Can you work these out from the model? Positions are in its coordinate system, mm. A direction names the side the tool comes from. Coordinates: 2 decimals unless noted, no trailing zeros. Order: outer loops, then holes, each group sorted by start corner. A loop starts at its lowest first (then second) coordinate and runs counter-clockwise, first axis right, second up. Notation, with made-up numbers: (48, 85.5) -> (89, 85.5) arc R27 ccw to (89, 103.5) -> close; hole circle Ø1 at (-9.5, 3). An arc over 180 degrees is marked (long way). Answer in a Markdown table with one row per item. Add a question column.
1. On a 3-axis mill with a long thin cutter (end or side, diameter ignored), from which of +Z, -Z, +X, -X, +Y, -Y can I reach the whole of each face in a straight line? I mean faces 1 (the face through (-160, -1, 65)), 2 (the face through (-2, 85, 65)), 3 (the face through (-155.49, -80.72, 65.35)), 4 (the face through (160, -1, 65)). Say none if no direction works.
2. If I drill on line 1 along X through (y, z) = (-57.5, 39.5); line 2 along Z through (x, y) = (225, 83); line 3 along Y through (x, z) = (17, 62), over which ranges is the centre line in solid material (lowest first)? Write a range as [from, to].
3. Will these pins go through, and if not, where does the flat tip stop? pin 1 (4 mm diameter, centred on x = 47.5, y = -89.5, fed in from +Z); pin 2 (15 mm diameter, centred on y = 32, z = 63.5, fed in from +X); pin 3 (8 mm diameter, centred on x = 159.5, z = 72.5, fed in from -Y).
4. Imagine slicing it at A-A on y = -1. Write out the boundary of the cut face in (x, z), plus the area to 3 significant figures.
5. Imagine slicing it at C-C on x = 75. Write out the boundary of the cut face in (y, z), plus the area to 3 significant figures.
6. Imagine slicing it at B-B on z = 57.5. Write out the boundary of the cut face in (x, y), plus the area to 3 significant figures.
7. Imagine slicing it at D-D on x = 214. Write out the boundary of the cut face in (y, z).
from build123d import *

# Parameters (mm, degrees)
F0_W     = 500
F0_H     = 250
F1_DEPTH = 25
F2_W     = 320
F2_H     = 170
F3_DEPTH = 80
F4_R     = 15


with BuildPart() as f1:
    # F0 (on Top) → F1 (new body, symmetric)
    with BuildSketch(Plane.XY):
        Rectangle(F0_W, F0_H)
    extrude(amount=F1_DEPTH, both=True)

    # F2 (on face) → F3 (join)
    with BuildSketch(Plane.XY.offset(25)):
        Rectangle(F2_W, F2_H)
    extrude(amount=F3_DEPTH)

    # F4
    f4_edges = [f1.edges().sort_by_distance(p)[0] for p in [
        (0, -85, 105),
        (-160, 0, 105),
        (160, 0, 105),
        (-160, -85, 65),
        (-160, 85, 65),
        (160, -85, 65),
        (0, 85, 105),
        (160, 85, 65),
        (0, -85, 25),
        (-160, 0, 25),
        (160, 0, 25),
        (0, 85, 25),
    ]]
    fillet(f4_edges, radius=F4_R)


solid = f1.part
Answers follow:
| question | item | result |
|---|---|---|
| 1 | face 1 | +Z, -X, +Y, -Y |
| 1 | face 2 | +Z, +X, -X, +Y |
| 1 | face 3 | +Z, -X, -Y |
| 1 | face 4 | +Z, +X, +Y, -Y |
| 2 | line 1 | x = [-160.01, 160.01] |
| 2 | line 2 | z = [-25, 25] |
| 2 | line 3 | y = [-85, 85] |
| 3 | pin 1 | stops at z = 31.71 |
| 3 | pin 2 | stops at x = 160 |
| 3 | pin 3 | stops at y = -80.71 |
| 4 | outline | (-250, -25) -> (250, -25) -> (250, 25) -> (175, 25) arc R15 cw to (160, 40) -> (160, 90) arc R15 ccw to (145, 105) -> (-145, 105) arc R15 ccw to (-160, 90) -> (-160, 40) arc R15 cw to (-175, 25) -> (-250, 25) -> close |
| 4 | area | 50,600 mm² |
| 5 | outline | (-125, -25) -> (125, -25) -> (125, 25) -> (100, 25) arc R15 cw to (85, 40) -> (85, 90) arc R15 ccw to (70, 105) -> (-70, 105) arc R15 ccw to (-85, 90) -> (-85, 40) arc R15 cw to (-100, 25) -> (-125, 25) -> close |
| 5 | area | 26,100 mm² |
| 6 | outline | (-160, -70) arc R15 ccw to (-145, -85) -> (145, -85) arc R15 ccw to (160, -70) -> (160, 70) arc R15 ccw to (145, 85) -> (-145, 85) arc R15 ccw to (-160, 70) -> close |
| 6 | area | 54,200 mm² |
| 7 | outline | (-125, -25) -> (125, -25) -> (125, 25) -> (-125, 25) -> close |
